Answer from the drawing. Dimensions are ordinates in mm from the lowest x, y and z of the part. A direction names the side the tool comes from. Give positions to 0.01 mm unless a question says otherwise; leave off trailing zeros. Order: outer loops, then holes, each group sorted by start corner. A loop starts at its lowest first (then second) coordinate and runs counter-clockwise, first axis right, second up.
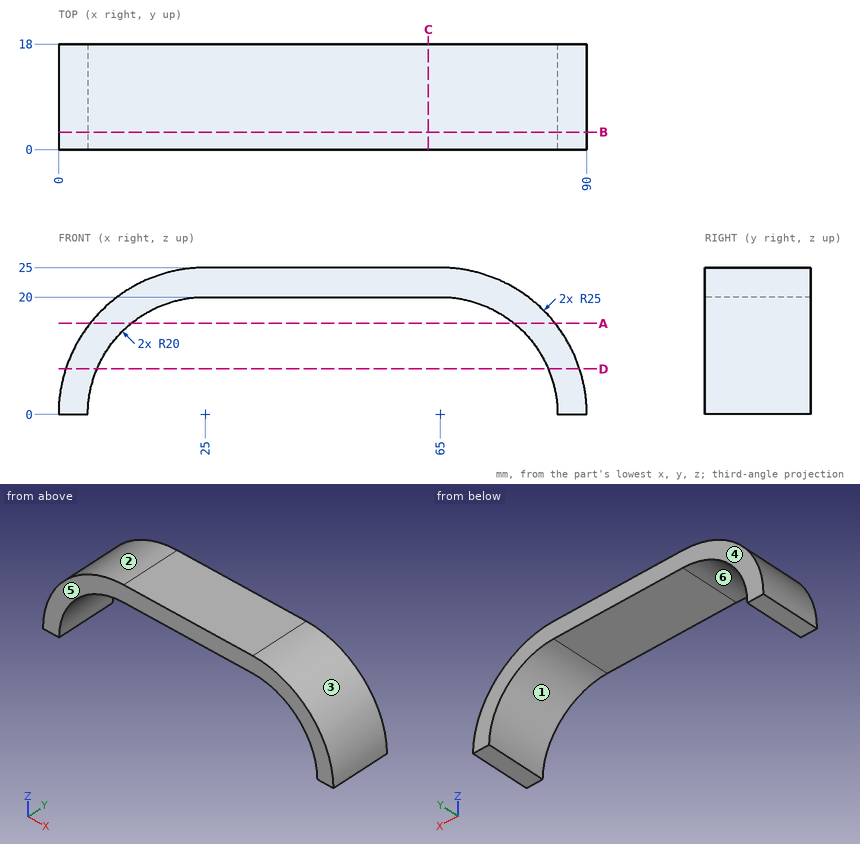
1. The part is cut by section A-A (z = 15.5). Write down the section's boundary in (x, y).
Findings below:
outline: (5.38, 0) - (12.36, 0) - (12.36, 18) - (5.38, 18) - close; (77.64, 0) - (84.62, 0) - (84.62, 18) - (77.64, 18) - close
2. The part is cut by section C-C (x = 63). Write down the section's boundary in (y, z), then the cut area to 3 significant figures.
Findings below:
outline: (0, 20) - (18, 20) - (18, 25) - (0, 25) - close
area: 90.0 mm2
3. The mould has two halves that part along X. Classify the marked faces 1, 2, 3 and 4: pulls with the +X half, pulls with the -X half, needs draft (parallel to the pull), parting line crosses it, or undercut.
Findings below:
face 1: undercut
face 2: pulls with the -X half
face 3: pulls with the +X half
face 4: needs draft
4. The part is cut by section B-B (y = 3). Write down the section's boundary in (x, z).
Findings below:
outline: (0, 0) - (5, 0) arc R20 cw to (25, 20) - (65, 20) arc R20 cw to (85, 0) - (90, 0) arc R25 ccw to (65, 25) - (25, 25) arc R25 ccw to start
5. Straight lines are drawn through the part: probe 1 along Z at (x, y) = (32.5, 5.5); probe 2 along X at (y, z) = (9.5, 17.5); probe 3 along X at (y, z) = (8.5, 18.5). For each, find the intervals that lie inside material, in ascending order.
Findings below:
probe 1: z = 20 to 25
probe 2: x = 7.15 to 15.32, 74.68 to 82.85
probe 3: x = 8.18 to 17.4, 72.6 to 81.82
6. Which of the six approach directions +Z, -Z, +X, -X, +Y, -Y give full straight-line access (tool end or side, diameter ignored) to the marked faces 5 and 6?
Findings below:
face 5: +Z, -Z, +X, -X, -Y
face 6: -Z, +Y, -Y
7. The part is cut by section D-D (z = 7.75). Write down the section's boundary in (x, y).
Findings below:
outline: (1.23, 0) - (6.56, 0) - (6.56, 18) - (1.23, 18) - close; (83.44, 0) - (88.77, 0) - (88.77, 18) - (83.44, 18) - close
8. Given P1, Ø10, axis at y = 5, z = 22, coming from the +X side; P2, Ø2, axis at x = 11, y = 9.5, coming from the +Z side; P3, Ø4, axis at y = 3.5, z = 16, coming from the +X side, each flat-ended and moving along its own axis, determine where each tip first touches the part or whether it passes through.
Findings below:
P1: stops at x = 83.33
P2: stops at z = 21.35
P3: stops at x = 85.71
